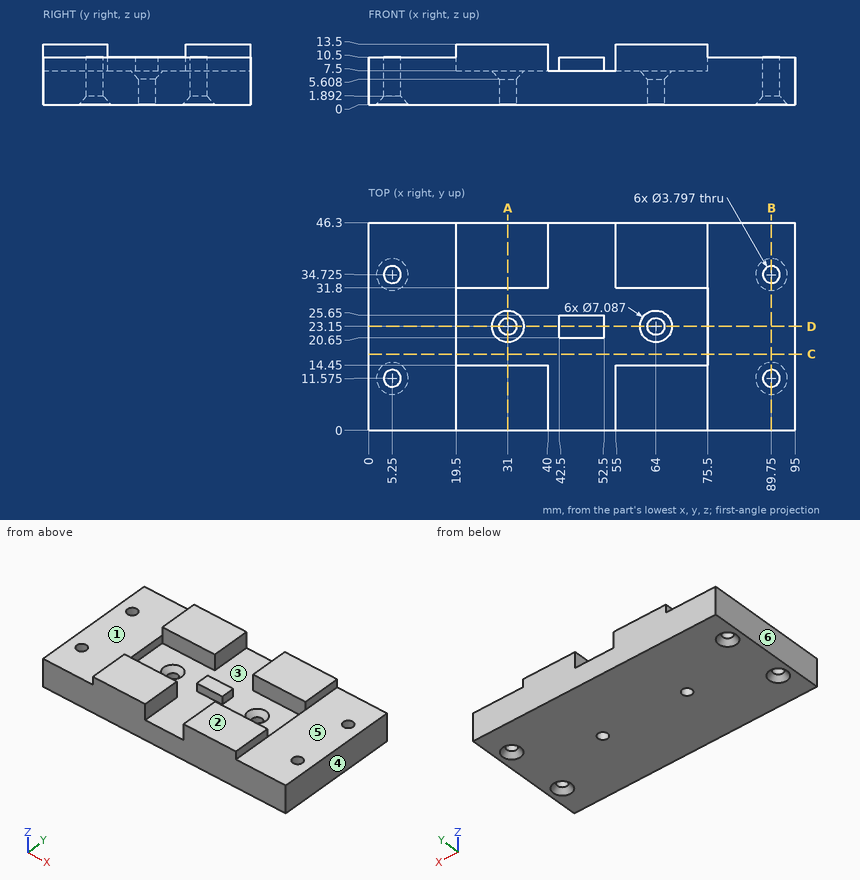
Answer from the drawing. Dimensions are ordinates in mm from the lowest x, y and z of the part. A direction names the side the tool comes from. Give positions to 0.01 mm unless a question says otherwise; leave off trailing zeros. Loops run counter-clockwise (first coordinate to the right, second up) from the corner with the lowest first, then second, coordinate; pieces in that order, holes last. Notation, with made-up numbers: (66, 70) - (119, 70) arc R23 ccw to (119, 106) - close; hole circle Ø1 at (10, 61.5). An arc over 180 degrees is marked (long way). Write each question's results on one line, items separated by ' | '.
1. Consider probe 1 along Y at (x, z) = (89.5, 3.75); probe 2 along X at (y, z) = (23.15, 2.4); probe 3 along X at (y, z) = (35, 5.75). Determine where each line is inside the solid, lowest interval first. Write a range as from..to.
Resolved:
probe 1: y = 0..9.69, 13.46..32.84, 36.61..46.3 | probe 2: x = 0..29.1, 32.9..62.1, 65.9..95 | probe 3: x = 0..3.37, 7.13..87.87, 91.63..95
2. Find section D-D, the plane y = 23.15. Write down the section's boundary in (x, z).
Resolved:
outline: (0, 0) - (29.1, 0) - (29.1, 5.61) - (27.46, 7.5) - (19.5, 7.5) - (19.5, 10.5) - (0, 10.5) - close; (32.9, 0) - (62.1, 0) - (62.1, 5.61) - (60.46, 7.5) - (52.5, 7.5) - (52.5, 10.5) - (42.5, 10.5) - (42.5, 7.5) - (34.54, 7.5) - (32.9, 5.61) - close; (65.9, 0) - (95, 0) - (95, 10.5) - (75.5, 10.5) - (75.5, 7.5) - (67.54, 7.5) - (65.9, 5.61) - close
3. Flat-ended cylindrical pins translate along their axes: P1, Ø1.8, axis at y = 7, z = 11.5, coming from the -X side; P2, Ø4.5, axis at x = 89.75, y = 34.725, coming from the +Z side; P3, Ø6, axis at x = 64, y = 23.15, coming from the +Z side (1 decimal). Find the tip coordinate at first contact, or state that the pin passes through.
Resolved:
P1: stops at x = 19.5 | P2: stops at z = 10.5 | P3: stops at z = 6.9
4. Find section C-C, the plane y = 17. Write down the section's boundary in (x, z).
Resolved:
outline: (0, 0) - (95, 0) - (95, 10.5) - (75.5, 10.5) - (75.5, 7.5) - (19.5, 7.5) - (19.5, 10.5) - (0, 10.5) - close
5. Which of the six approach directions +Z, -Z, +X, -X, +Y, -Y give full straight-line access (tool end or side, diameter ignored) to the marked faces 1 and 2?
Resolved:
face 1: +Z, -X, +Y, -Y | face 2: +Z, +X, -X, +Y, -Y
6. Find section B-B, the plane x = 89.75. Write down the section's boundary in (y, z).
Resolved:
outline: (0, 0) - (8.03, 0) - (9.68, 1.89) - (9.68, 10.5) - (0, 10.5) - close; (13.47, 1.89) - (15.12, 0) - (31.18, 0) - (32.83, 1.89) - (32.83, 10.5) - (13.47, 10.5) - close; (36.62, 1.89) - (38.27, 0) - (46.3, 0) - (46.3, 10.5) - (36.62, 10.5) - close
7. For a pull along X with two mould halves and no side action, classify the marked faces 3, 4, 5 and 6 as +X half, -X half, draft (parallel to the pull), parting line (faces both ways), or undercut.
Resolved:
face 3: undercut | face 4: +X half | face 5: draft | face 6: -X half
8. Find section A-A, the plane x = 31. Write down the section's boundary in (y, z), then the cut area to 3 significant figures.
Resolved:
outline: (0, 0) - (21.25, 0) - (21.25, 5.61) - (19.61, 7.5) - (14.45, 7.5) - (14.45, 13.5) - (0, 13.5) - close; (25.05, 0) - (46.3, 0) - (46.3, 13.5) - (31.8, 13.5) - (31.8, 7.5) - (26.69, 7.5) - (25.05, 5.61) - close | area: 489 mm^2
